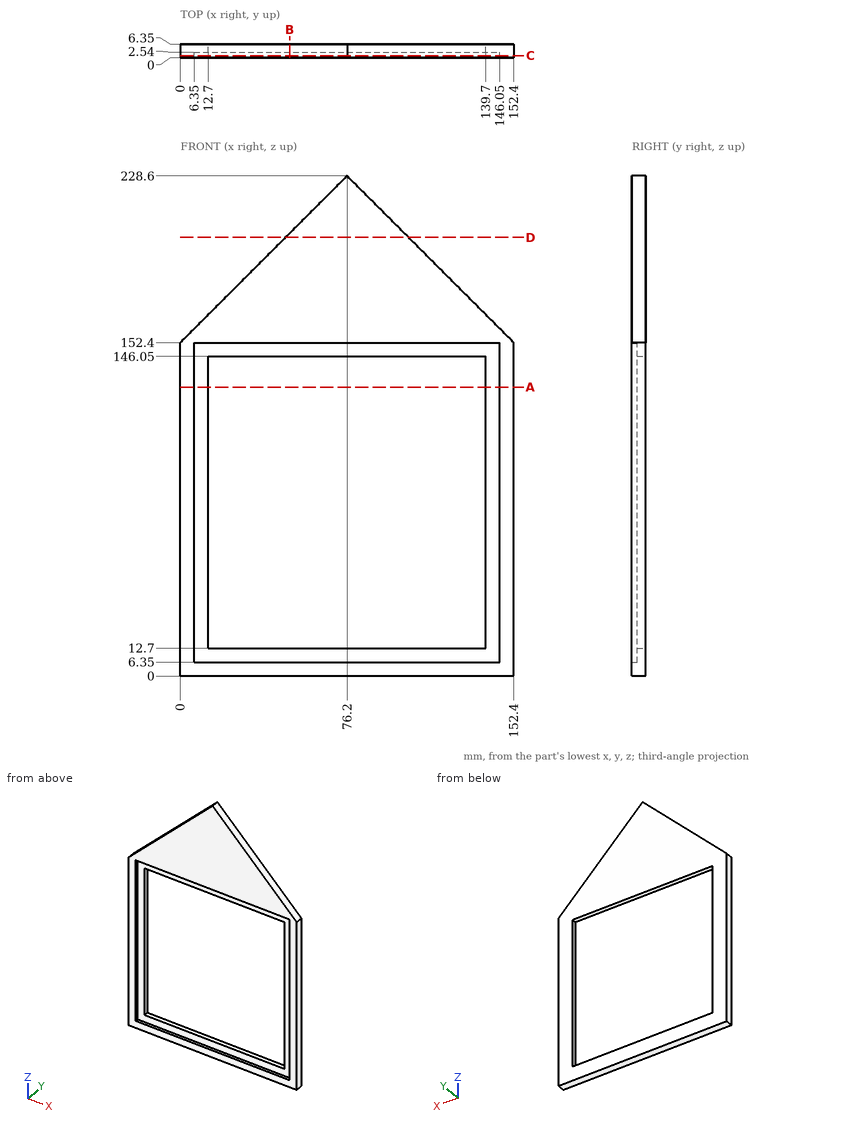
Design review of the part shown in the three views and the two pictorial views. Dimensions are in mm from the part's minimum x, y and z. Coordinates: 2 decimals unless noted, no trailing zeros. Loops run counter-clockwise (first coordinate to the right, second up) from the corner with the lowest first, then second, coordinate; pieces in that order, holes last.
Q1. We need section C-C on y = 1. State the section outline as (x, z) points.
Reported:
outline: (0, 0) - (152.4, 0) - (152.4, 152.4) - (76.2, 228.6) - (0, 152.4) - close; hole (6.35, 6.35) - (146.05, 6.35) - (146.05, 152.4) - (6.35, 152.4) - close
Q2. We need section D-D on z = 200.5. State the section outline as (x, y) points, and give its area (3 significant figures).
Reported:
outline: (48.1, 0) - (104.3, 0) - (104.3, 6.35) - (48.1, 6.35) - close
area: 357 mm2
Q3. For pin 1 (0.8 mm diameter, centred on x = 104.5, y = 1, fed in from +Z); pin 2 (1.9 mm diameter, centred on x = 63.5, y = 4.5, fed in from +Z); pin 3 (8 mm diameter, centred on x = 134, z = 129.5, fed in from -Y), all flat-tipped, find the tip position at first contact; note any pin that passes through.
Reported:
pin 1: stops at z = 200.7
pin 2: stops at z = 216.85
pin 3: passes through
Q4. To check wall thickness, follow line 1 (X direction, y = 5.5, z = 62.5); line 2 (X direction, y = 2, z = 83.5); line 3 (Z direction, x = 34.5, y = 5). State the ranges of each line that lie inside material, in increasing order.
Reported:
line 1: x = 0 to 12.7, 139.7 to 152.4
line 2: x = 0 to 6.35, 146.05 to 152.4
line 3: z = 0 to 12.7, 146.05 to 186.9
Q5. We need section B-B on x = 50. State the section outline as (y, z) points.
Reported:
outline: (0, 0) - (6.35, 0) - (6.35, 12.7) - (2.54, 12.7) - (2.54, 6.35) - (0, 6.35) - close; (0, 152.4) - (2.54, 152.4) - (2.54, 146.05) - (6.35, 146.05) - (6.35, 202.4) - (0, 202.4) - close
Q6. We need section A-A on z = 132. State the section outline as (x, y) points.
Reported:
outline: (0, 0) - (6.35, 0) - (6.35, 2.54) - (12.7, 2.54) - (12.7, 6.35) - (0, 6.35) - close; (139.7, 2.54) - (146.05, 2.54) - (146.05, 0) - (152.4, 0) - (152.4, 6.35) - (139.7, 6.35) - close
